Input: part model. Units: mm. Frame: model coordinates. Face numbers are marked on the shaded views. A direction names the side the tool comes from. Round coordinates to 2 decimals unless told otherwise and drop trailing zeros. Loops run counter-clockwise (first coordinate to the right, second up) from the corner with the lowest first, then second, coordinate; pieces in that order, holes last. Notation, with made-up numbers: (-34.5, -25.5) -> (23.5, -25.5) arc R28 ccw to (23.5, 11.5) -> close; hole circle Ø10 at (-32, -31). An arc over 180 degrees is marked (long way). One line per question, with ' | ' between items. Start each with the question number.
Q1. Cut plane A-A on x = 5. Return loops of the section in (y, z).
Q2. Material intervals for L1, parallel to Y at x = 5, z = 6; L2, parallel to Z at x = -9.5, y = -6.5; L3, parallel to X at y = -9.5, z = 16, sorted ascending.
Q3. Mould query, pull axis X, two halves, no side actions, for the marked faces 4, 5 and 6. Classes: pulls with the +X half, pulls with the -X half, needs draft (parallel to the pull), parting line crosses it, or undercut.
Q4. Cut plane B-B on x = -21. Return loops of the section in (y, z).
Q5. Cut plane C-C on y = -5. Return loops of the section in (x, z), and give its area (3 significant figures).
Q6. Contact query for flat-ended pins moving along their axis: P1, Ø5, axis at x = -21, z = 19, coming from the -Y side; P2, Ø6, axis at x = 13, y = 11, coming from the +Z side; P3, Ø3, axis at y = 0, z = 21, coming from the +X side. Output: stop coordinate, or through.
Q7. Cut plane D-D on z = 20. Return loops of the section in (x, y), and give its area (3 significant figures).
Q8. Access query for the marked faces 1, 2 and 3. Directions: +Z, -Z, +X, -X, +Y, -Y. A direction counts if a zero-diameter tool reaches every point of the face in a straight line with its end or side. Return the directions, or none.
from build123d import *

# Parameters (mm, degrees)
PAD001_DEPTH = 10
SKETCH_R     = 6
PAD_DEPTH    = 11.5
PAD002_DEPTH = 10


with BuildPart() as lateral_i:
    # Sketch001 → Pad001 (new body)
    with BuildSketch(Plane.YZ.offset(-27)):
        Polygon((27, 0), (27, 44.5), (13, 44.5), (-12.1, 24.7), (-12.1, 0), align=None)
    extrude(amount=PAD001_DEPTH)


with BuildPart() as base:
    # Sketch → Pad (new body)
    with BuildSketch(Plane.XY):
        Polygon((-27, 27), (27, 27), (27, -8), (8, -27), (-27, -27), align=None)
        with Locations((5, -5)):
            Circle(SKETCH_R, mode=Mode.SUBTRACT)
    extrude(amount=PAD_DEPTH)


with BuildPart() as pieza_laterales:
    # Sketch002 → Pad002 (new body)
    with BuildSketch(Plane(origin=(5, 27, 0), x_dir=(1, 0, 0), z_dir=(0, -1, 0))):
        Polygon((22, 11.5), (22, 16.5), (-22, 36.5), (-22, 11.5), align=None)
    extrude(amount=PAD002_DEPTH)

    # Fusion: union Lateral-I, Base
    add(lateral_i.part)
    add(base.part)


solid = pieza_laterales.part
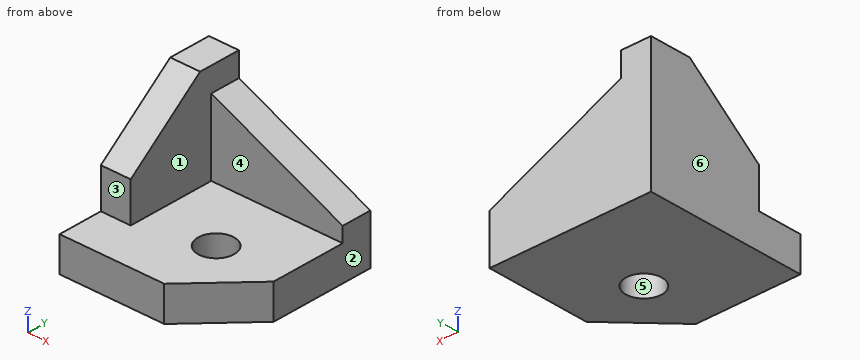
Results:
1) outline: (-27, 0) -> (-11, 0) -> (-11, 11.5) -> (-27, 11.5) -> close; (1, 0) -> (27, 0) -> (27, 26.5) -> (17, 26.5) -> (17, 11.5) -> (1, 11.5) -> close
2) L1: -27 to -11, 1 to 27 | L2: 0 to 11.5 | L3: -27 to -17
3) face 4: needs draft | face 5: undercut | face 6: pulls with the -X half
4) outline: (-27, 0) -> (27, 0) -> (27, 44.5) -> (13, 44.5) -> (-12.1, 24.7) -> (-12.1, 11.5) -> (-27, 11.5) -> close
5) outline: (-27, 0) -> (-1, 0) -> (-1, 11.5) -> (-17, 11.5) -> (-17, 30.3) -> (-27, 30.3) -> close; (11, 0) -> (27, 0) -> (27, 11.5) -> (11, 11.5) -> close | area: 671 mm^2
6) P1: y = -12.1 | P2: z = 11.5 | P3: x = -17
7) outline: (-27, -12.1) -> (-17, -12.1) -> (-17, 17) -> (19.3, 17) -> (19.3, 27) -> (-27, 27) -> close | area: 754 mm^2
8) face 1: +Z, +X, -Y | face 2: +Z, -Z, +X, +Y, -Y | face 3: +Z, +X, -X, -Y
